Verification items for the finished model (mm, model axes). Coordinates: 2 decimals unless noted, no trailing zeros. Order: outer loops, then holes, each group sorted by start corner. A loop starts at its lowest first (then second) coordinate and runs counter-clockwise, first axis right, second up. Notation, with made-up numbers: M 77.25,20.25 L 120.25,20.25 A19 cw 120.25,31.25 Z; hole C 3,67.5 d11. An arc over 180 degrees is marked long. Write item = value, one per line.
```python
from build123d import *

# Parameters (mm, degrees)
F0_R     = 5.45
F1_DEPTH = 0.2


with BuildPart() as f1:
    # F0 (on Top) → F1 (new body)
    with BuildSketch(Plane.XY):
        Circle(F0_R)
        with BuildLine():
            ThreePointArc((4.993959, 0.245708), (4.99849, 0.122891), (5, 0))
            ThreePointArc((5, 0), (4.99849, -0.122891), (4.993959, -0.245708))
            ThreePointArc((4.993959, -0.245708), (4.957224, -0.652631), (4.887388, -1.055196))
            ThreePointArc((4.887388, -1.055196), (4.829629, -1.294095), (4.7602, -1.529867))
            ThreePointArc((4.7602, -1.529867), (4.619398, -1.913417), (4.447749, -2.28419))
            ThreePointArc((4.447749, -2.28419), (4.330127, -2.5), (4.202042, -2.709769))
            ThreePointArc((4.202042, -2.709769), (3.966767, -3.043807), (3.705004, -3.357521))
            ThreePointArc((3.705004, -3.357521), (3.535534, -3.535534), (3.357521, -3.705004))
            ThreePointArc((3.357521, -3.705004), (3.043807, -3.966767), (2.709769, -4.202042))
            ThreePointArc((2.709769, -4.202042), (2.5, -4.330127), (2.28419, -4.447749))
            ThreePointArc((2.28419, -4.447749), (1.913417, -4.619398), (1.529867, -4.7602))
            ThreePointArc((1.529867, -4.7602), (1.294095, -4.829629), (1.055196, -4.887388))
            ThreePointArc((1.055196, -4.887388), (0.652631, -4.957224), (0.245708, -4.993959))
            ThreePointArc((0.245708, -4.993959), (0, -5), (-0.245708, -4.993959))
            ThreePointArc((-0.245708, -4.993959), (-0.652631, -4.957224), (-1.055196, -4.887388))
            ThreePointArc((-1.055196, -4.887388), (-1.294095, -4.829629), (-1.529867, -4.7602))
            ThreePointArc((-1.529867, -4.7602), (-1.913417, -4.619398), (-2.28419, -4.447749))
            ThreePointArc((-2.28419, -4.447749), (-2.5, -4.330127), (-2.709769, -4.202042))
            ThreePointArc((-2.709769, -4.202042), (-3.043807, -3.966767), (-3.357521, -3.705004))
            ThreePointArc((-3.357521, -3.705004), (-3.535534, -3.535534), (-3.705004, -3.357521))
            ThreePointArc((-3.705004, -3.357521), (-3.966767, -3.043807), (-4.202042, -2.709769))
            ThreePointArc((-4.202042, -2.709769), (-4.330127, -2.5), (-4.447749, -2.28419))
            ThreePointArc((-4.447749, -2.28419), (-4.619398, -1.913417), (-4.7602, -1.529867))
            ThreePointArc((-4.7602, -1.529867), (-4.829629, -1.294095), (-4.887388, -1.055196))
            ThreePointArc((-4.887388, -1.055196), (-4.957224, -0.652631), (-4.993959, -0.245708))
            ThreePointArc((-4.993959, -0.245708), (-5, 0), (-4.993959, 0.245708))
            ThreePointArc((-4.993959, 0.245708), (-4.957224, 0.652631), (-4.887388, 1.055196))
            ThreePointArc((-4.887388, 1.055196), (-4.829629, 1.294095), (-4.7602, 1.529867))
            ThreePointArc((-4.7602, 1.529867), (-4.619398, 1.913417), (-4.447749, 2.28419))
            ThreePointArc((-4.447749, 2.28419), (-4.330127, 2.5), (-4.202042, 2.709769))
            ThreePointArc((-4.202042, 2.709769), (-3.966767, 3.043807), (-3.705004, 3.357521))
            ThreePointArc((-3.705004, 3.357521), (-3.535534, 3.535534), (-3.357521, 3.705004))
            ThreePointArc((-3.357521, 3.705004), (-3.043807, 3.966767), (-2.709769, 4.202042))
            ThreePointArc((-2.709769, 4.202042), (-2.5, 4.330127), (-2.28419, 4.447749))
            ThreePointArc((-2.28419, 4.447749), (-1.913417, 4.619398), (-1.529867, 4.7602))
            ThreePointArc((-1.529867, 4.7602), (-1.294095, 4.829629), (-1.055196, 4.887388))
            ThreePointArc((-1.055196, 4.887388), (-0.652631, 4.957224), (-0.245708, 4.993959))
            ThreePointArc((-0.245708, 4.993959), (0, 5), (0.245708, 4.993959))
            ThreePointArc((0.245708, 4.993959), (0.652631, 4.957224), (1.055196, 4.887388))
            ThreePointArc((1.055196, 4.887388), (1.294095, 4.829629), (1.529867, 4.7602))
            ThreePointArc((1.529867, 4.7602), (1.913417, 4.619398), (2.28419, 4.447749))
            ThreePointArc((2.28419, 4.447749), (2.5, 4.330127), (2.709769, 4.202042))
            ThreePointArc((2.709769, 4.202042), (3.043807, 3.966767), (3.357521, 3.705004))
            ThreePointArc((3.357521, 3.705004), (3.535534, 3.535534), (3.705004, 3.357521))
            ThreePointArc((3.705004, 3.357521), (3.966767, 3.043807), (4.202042, 2.709769))
            ThreePointArc((4.202042, 2.709769), (4.330127, 2.5), (4.447749, 2.28419))
            ThreePointArc((4.447749, 2.28419), (4.619398, 1.913417), (4.7602, 1.529867))
            ThreePointArc((4.7602, 1.529867), (4.829629, 1.294095), (4.887388, 1.055196))
            ThreePointArc((4.887388, 1.055196), (4.957224, 0.652631), (4.993959, 0.245708))
        make_face(mode=Mode.SUBTRACT)
        with BuildLine():
            Line((-2.196215, 3.803956), (-2.28419, 4.447749))
            ThreePointArc((-2.28419, 4.447749), (-2.5, 4.330127), (-2.709769, 4.202042))
            Line((-2.709769, 4.202042), (-2.196215, 3.803956))
        make_face()
        with BuildLine():
            Line((-1.136845, 4.242762), (-1.055196, 4.887388))
            ThreePointArc((-1.055196, 4.887388), (-1.294095, 4.829629), (-1.529867, 4.7602))
            Line((-1.529867, 4.7602), (-1.136845, 4.242762))
        make_face()
        with BuildLine():
            Line((-3.105917, 3.105917), (-3.357521, 3.705004))
            ThreePointArc((-3.357521, 3.705004), (-3.535534, 3.535534), (-3.705004, 3.357521))
            Line((-3.705004, 3.357521), (-3.105917, 3.105917))
        make_face()
        with BuildLine():
            Line((-3.803956, 2.196215), (-4.202042, 2.709769))
            ThreePointArc((-4.202042, 2.709769), (-4.330127, 2.5), (-4.447749, 2.28419))
            Line((-4.447749, 2.28419), (-3.803956, 2.196215))
        make_face()
        with BuildLine():
            Line((-4.242762, 1.136845), (-4.7602, 1.529867))
            ThreePointArc((-4.7602, 1.529867), (-4.829629, 1.294095), (-4.887388, 1.055196))
            Line((-4.887388, 1.055196), (-4.242762, 1.136845))
        make_face()
        with BuildLine():
            Line((-4.39243, 0), (-4.993959, 0.245708))
            ThreePointArc((-4.993959, 0.245708), (-5, 0), (-4.993959, -0.245708))
            Line((-4.993959, -0.245708), (-4.39243, 0))
        make_face()
        with BuildLine():
            ThreePointArc((-4.887388, -1.055196), (-4.829629, -1.294095), (-4.7602, -1.529867))
            Line((-4.7602, -1.529867), (-4.242762, -1.136845))
            Line((-4.242762, -1.136845), (-4.887388, -1.055196))
        make_face()
        with BuildLine():
            ThreePointArc((-4.447749, -2.28419), (-4.330127, -2.5), (-4.202042, -2.709769))
            Line((-4.202042, -2.709769), (-3.803956, -2.196215))
            Line((-3.803956, -2.196215), (-4.447749, -2.28419))
        make_face()
        with BuildLine():
            ThreePointArc((-3.705004, -3.357521), (-3.535534, -3.535534), (-3.357521, -3.705004))
            Line((-3.357521, -3.705004), (-3.105917, -3.105917))
            Line((-3.105917, -3.105917), (-3.705004, -3.357521))
        make_face()
        with BuildLine():
            ThreePointArc((-2.709769, -4.202042), (-2.5, -4.330127), (-2.28419, -4.447749))
            Line((-2.28419, -4.447749), (-2.196215, -3.803956))
            Line((-2.196215, -3.803956), (-2.709769, -4.202042))
        make_face()
        with BuildLine():
            ThreePointArc((-1.529867, -4.7602), (-1.294095, -4.829629), (-1.055196, -4.887388))
            Line((-1.055196, -4.887388), (-1.136845, -4.242762))
            Line((-1.136845, -4.242762), (-1.529867, -4.7602))
        make_face()
        with BuildLine():
            ThreePointArc((-0.245708, -4.993959), (0, -5), (0.245708, -4.993959))
            Line((0.245708, -4.993959), (0, -4.39243))
            Line((0, -4.39243), (-0.245708, -4.993959))
        make_face()
        with BuildLine():
            ThreePointArc((1.055196, -4.887388), (1.294095, -4.829629), (1.529867, -4.7602))
            Line((1.529867, -4.7602), (1.136845, -4.242762))
            Line((1.136845, -4.242762), (1.055196, -4.887388))
        make_face()
        with BuildLine():
            ThreePointArc((2.28419, -4.447749), (2.5, -4.330127), (2.709769, -4.202042))
            Line((2.709769, -4.202042), (2.196215, -3.803956))
            Line((2.196215, -3.803956), (2.28419, -4.447749))
        make_face()
        with BuildLine():
            ThreePointArc((3.357521, -3.705004), (3.535534, -3.535534), (3.705004, -3.357521))
            Line((3.705004, -3.357521), (3.105917, -3.105917))
            Line((3.105917, -3.105917), (3.357521, -3.705004))
        make_face()
        with BuildLine():
            ThreePointArc((4.202042, -2.709769), (4.330127, -2.5), (4.447749, -2.28419))
            Line((4.447749, -2.28419), (3.803956, -2.196215))
            Line((3.803956, -2.196215), (4.202042, -2.709769))
        make_face()
        with BuildLine():
            ThreePointArc((4.7602, -1.529867), (4.829629, -1.294095), (4.887388, -1.055196))
            Line((4.887388, -1.055196), (4.242762, -1.136845))
            Line((4.242762, -1.136845), (4.7602, -1.529867))
        make_face()
        with BuildLine():
            ThreePointArc((4.993959, -0.245708), (4.99849, -0.122891), (5, 0))
            ThreePointArc((5, 0), (4.99849, 0.122891), (4.993959, 0.245708))
            Line((4.993959, 0.245708), (4.39243, 0))
            Line((4.39243, 0), (4.993959, -0.245708))
        make_face()
        with BuildLine():
            Line((4.242762, 1.136845), (4.887388, 1.055196))
            ThreePointArc((4.887388, 1.055196), (4.829629, 1.294095), (4.7602, 1.529867))
            Line((4.7602, 1.529867), (4.242762, 1.136845))
        make_face()
        with BuildLine():
            Line((3.803956, 2.196215), (4.447749, 2.28419))
            ThreePointArc((4.447749, 2.28419), (4.330127, 2.5), (4.202042, 2.709769))
            Line((4.202042, 2.709769), (3.803956, 2.196215))
        make_face()
        with BuildLine():
            Line((3.105917, 3.105917), (3.705004, 3.357521))
            ThreePointArc((3.705004, 3.357521), (3.535534, 3.535534), (3.357521, 3.705004))
            Line((3.357521, 3.705004), (3.105917, 3.105917))
        make_face()
        with BuildLine():
            Line((2.196215, 3.803956), (2.709769, 4.202042))
            ThreePointArc((2.709769, 4.202042), (2.5, 4.330127), (2.28419, 4.447749))
            Line((2.28419, 4.447749), (2.196215, 3.803956))
        make_face()
        with BuildLine():
            Line((1.136845, 4.242762), (1.529867, 4.7602))
            ThreePointArc((1.529867, 4.7602), (1.294095, 4.829629), (1.055196, 4.887388))
            Line((1.055196, 4.887388), (1.136845, 4.242762))
        make_face()
        with BuildLine():
            Line((0, 4.39243), (0.245708, 4.993959))
            ThreePointArc((0.245708, 4.993959), (0, 5), (-0.245708, 4.993959))
            Line((-0.245708, 4.993959), (0, 4.39243))
        make_face()
    extrude(amount=F1_DEPTH)


solid = f1.part
```
Item 1: Scan lines: L1, parallel to X at y = 4, z = 0.1; L2, parallel to Y at x = -0.5, z = 0.05; L3, parallel to Y at x = -1.75, z = 0.15. Record each from-to range of solid material in increasing order. Write a range as from..to.
Report:
L1 = -3.7..-3, -2.45..-2.22, 2.22..2.45, 3..3.7
L2 = -5.43..-4.97, 4.97..5.43
L3 = -5.16..-4.68, 4.68..5.16
Item 2: Sectioned sample at A-A, the plane x = 3.5. Enter the section's corners in (y, z).
Report:
outline = M -4.18,0 L -3.27,0 L -3.27,0.2 L -4.18,0.2 Z; M 3.27,0 L 4.18,0 L 4.18,0.2 L 3.27,0.2 Z
